The model under review builds one solid part; all positions refer to its coordinate system, in mm. Face numbers are marked on the shaded views. A direction names the side the tool comes from. Give positions to 0.01 mm unless a question says otherwise; leave off trailing zeros. Order: outer loops, then holes, each group sorted by start corner. A loop starts at its lowest first (then second) coordinate and runs counter-clockwise, first axis right, second up. Notation, with made-up numbers: (-37, 66.25) -> (10, 66.25) arc R20 ccw to (10, 70.25) -> close; hole circle Ø11 at (35.25, 67.25). An arc over 180 degrees is marked (long way). Answer as a JSON object with one key per item and string values. Group by question number.
from build123d import *

# Parameters (mm, degrees)
CYLINDER_R           = 3
CYLINDER_DEPTH       = 10
CYLINDER_PITCH_ANGLE = -90
BOX032_W             = 54
BOX032_H             = 14
BOX032_DEPTH         = 15
BOX033_W             = 54
BOX033_H             = 16
BOX033_DEPTH         = 17
FILLET002_R          = 6.9
FILLET003_R          = 6.9
BOX_W                = 4
BOX_H                = 16
BOX_DEPTH            = 17


with BuildPart() as cylinder:
    # Cylinder → Cylinder (new body)
    with BuildSketch(Plane.XY):
        Circle(CYLINDER_R)
    extrude(amount=CYLINDER_DEPTH)


with BuildPart() as cylinder_1:
    # Cylinder pitch: moved
    add(cylinder.part.rotate(Axis((0, 0, 0), (0, 1, 0)), CYLINDER_PITCH_ANGLE))


with BuildPart() as cylinder_2:
    # Cylinder placement: moved
    add(cylinder_1.part.moved(Location((47, 7, -14))))


with BuildPart() as obj1:
    # Box032 → Box032 (new body)
    with BuildSketch(Plane(origin=(-9, 0, -21), x_dir=(1, 0, 0), z_dir=(0, 0, 1))):
        with Locations((27, 7)):
            Rectangle(BOX032_W, BOX032_H)
    extrude(amount=BOX032_DEPTH)


with BuildPart() as fillet003:
    # Box033 → Box033 (new body)
    with BuildSketch(Plane(origin=(-10, -1, -22), x_dir=(1, 0, 0), z_dir=(0, 0, 1))):
        with Locations((27, 8)):
            Rectangle(BOX033_W, BOX033_H)
    extrude(amount=BOX033_DEPTH)

    # Cut001: cut obj1
    add(obj1.part, mode=Mode.SUBTRACT)

    # Fillet002
    fillet002_edges = [fillet003.edges().sort_by_distance(p)[0] for p in [
        (17.5, 0, -21),
    ]]
    fillet(fillet002_edges, radius=FILLET002_R)

    # Fillet003
    fillet003_edges = [fillet003.edges().sort_by_distance(p)[0] for p in [
        (17.5, 14, -21),
    ]]
    fillet(fillet003_edges, radius=FILLET003_R)


with BuildPart() as cap:
    # Box → Box (new body)
    with BuildSketch(Plane(origin=(42, -1, -22), x_dir=(1, 0, 0), z_dir=(0, 0, 1))):
        with Locations((2, 8)):
            Rectangle(BOX_W, BOX_H)
    extrude(amount=BOX_DEPTH)

    # Cut002: cut Fillet003
    add(fillet003.part, mode=Mode.SUBTRACT)


with BuildPart() as cap_1:
    # Cut002 placement: moved
    add(cap.part.moved(Location((4, 0, 0))))

    # Cut003: cut Cylinder
    add(cylinder_2.part, mode=Mode.SUBTRACT)


with BuildPart() as cap_2:
    # Cut003 placement: moved
    add(cap_1.part.moved(Location((-4, 0, 0))))


solid = cap_2.part
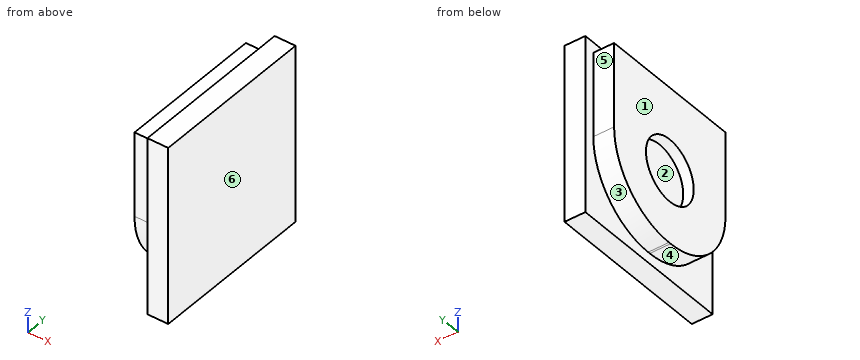
1. Take a section at B-B on z = -8.5. Give the boundary of the cut face in (x, y), plus the area to 3 significant figures.
2. Take a section at C-C on y = 7.75. Give the boundary of the cut face in (x, z), plus the area to 3 significant figures.
3. Machinability: for the marked faces 4, 5 and 6, which of the approach directions +Z, -Z, +X, -X, +Y, -Y give a long, thin tool a straight path to every point of the face, cutting with its end or side? Answer none if there is none.
4. Take a section at A-A on x = 42.55. Give the boundary of the cut face in (y, z).
5. Take a section at D-D on z = -11.5. Give the boundary of the cut face in (x, y).
6. For pin 1 (1.6 mm diameter, centred on x = 42.5, z = -9.5, fed in from +Y); pin 2 (1 mm diameter, centred on x = 43, y = 4.5, fed in from +Z), all flat-tipped, find the tip position at first contact; note any pin that passes through.
7. For probe 1 along Z at (x, y) = (42.35, 7); probe 2 along Y at (x, z) = (42.75, -14); probe 3 along X at (y, z) = (6.25, -13.5), list the stretches that pass through material, from the lowest coordinate up. Write a range as [from, to].
8. Draft analysis for pull direction Z (two halves, no side actions). For the marked faces 1, 2 and 3, state which applies: pulls with the +Z half, pulls with the -Z half, needs draft (parallel to the pull), parting line crosses it, or undercut.
Checks:
{
 "1": {"outline": "(42, 0) -> (44, 0) -> (44, -1) -> (46, -1) -> (46, 15) -> (44, 15) -> (44, 14) -> (42, 14) -> close", "area": "60.0 mm2"},
 "2": {"outline": "(42, -20.97) -> (44, -20.97) -> (44, -22) -> (46, -22) -> (46, -5) -> (44, -5) -> (44, -6) -> (42, -6) -> (42, -11.1) -> (43, -11.1) -> (43, -16.9) -> (42, -16.9) -> close", "area": "58.1 mm2"},
 "3": {"face 4": "-Z, -X, -Y", "face 5": "+Z, -Z, -X, +Y", "face 6": "+Z, -Z, +X, +Y, -Y"},
 "4": {"outline": "(0, -14.1) arc R6.9 ccw to (6.9, -21) -> (7.1, -21) arc R6.9 ccw to (14, -14.1) -> (14, -6) -> (0, -6) -> close; hole circle Ø6 at (7, -14)"},
 "5": {"outline": "(42, 0) -> (44, 0) -> (44, -1) -> (46, -1) -> (46, 15) -> (44, 15) -> (44, 14) -> (42, 14) -> (42, 8.66) -> (43, 8.66) -> (43, 5.34) -> (42, 5.34) -> close"},
 "6": {"pin 1": "stops at y = 14", "pin 2": "stops at z = -6"},
 "7": {"probe 1": "z = [-21, -17], [-11, -6]", "probe 2": "y = [0, 4], [10, 14]", "probe 3": "x = [43, 46]"},
 "8": {"face 1": "needs draft", "face 2": "undercut", "face 3": "pulls with the -Z half"}
}
